Drawing for the job (mm, zero at the part's lowest x, y, z). A direction names the side the tool comes from. Round coordinates to 2 decimals unless told otherwise and drop trailing zeros. Loops run counter-clockwise (first coordinate to the right, second up) from the corner with the lowest first, then second, coordinate; pieces in that order, holes last. Notation, with made-up numbers: M 70,46.5 L 113,46.5 A18 ccw 113,51.5 Z; hole C 87,56.5 d11. An arc over 180 degrees is marked long. Use a Markdown table: item, result. Add a question column.
Q1. Probe line 1 (Y direction, x = 60.5, z = 3.75) (1 decimal); line 2 (X direction, y = 74, z = 5) (1 decimal); line 3 (Y direction, x = 13.5, z = 5.5). List the from-to ranges inside material, lowest first. Write a range as from..to.
Q2. Cut at A-A (x = 36). Give the cut face in (y, z) (1 decimal), plus the area to 3 significant figures.
Q3. Pin check, flat tips, straight feed: pin 1 (3 mm diameter, centred on y = 59, z = 7, fed in from -X) (1 decimal); pin 2 (5 mm diameter, centred on x = 60.325, y = 40.64, fed in from -Z); pin 3 (5 mm diameter, centred on x = 7, z = 3.5, fed in from +Y); pin 4 (3 mm diameter, centred on x = 13.5, z = 5.5, fed in from +Y). Stop position of each tip, or through.
Q4. Tool access for the marked faces 1, 2 and 3: list every direction of +Z, -Z, +X, -X, +Y, -Y with a clear straight run to the whole face (end or side of a thin tool).
Q5. Cut at B-B (z = 8). State how many separate pieces and enclosed holes the cut face has, plus the area to 3 significant figures.
Q6. Mould opens along X. For the marked faces 4, 5 and 6 say: +X half, -X half, draft (parallel to the pull), parting line (faces both ways), or undercut.
Q7. Cut at C-C (y = 64.5). Give the cut face in (x, z) (1 decimal).
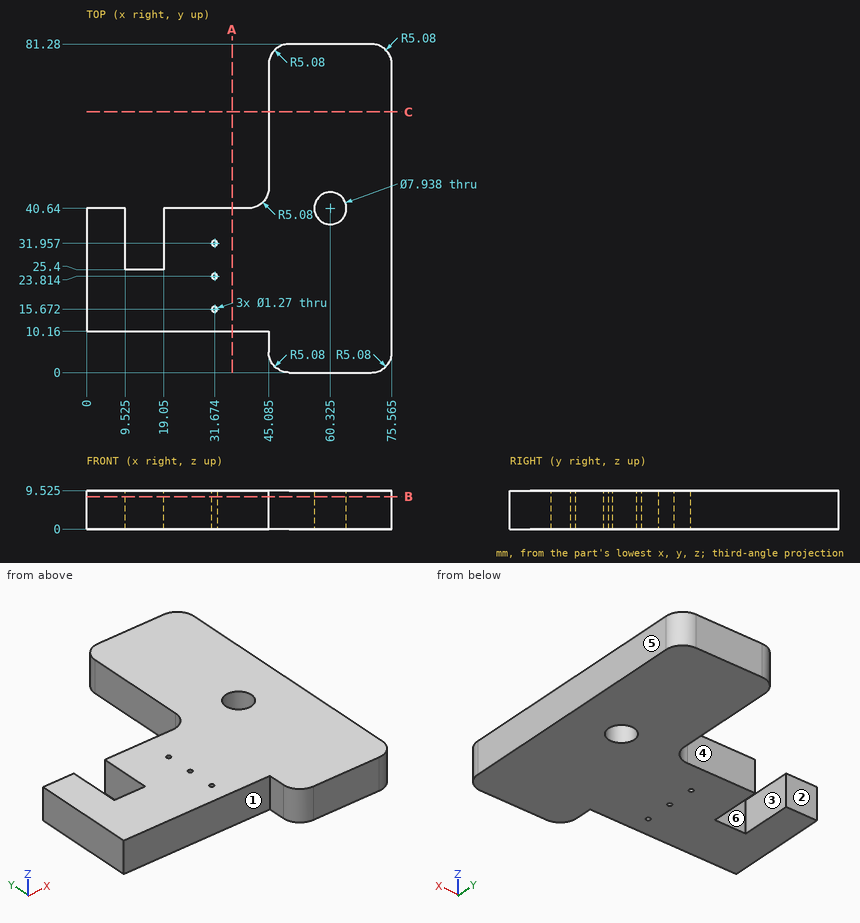
Checked values:
| question | item | result |
|---|---|---|
| 1 | line 1 | y = 0..36.7, 44.6..81.3 |
| 1 | line 2 | x = 45.1..75.6 |
| 1 | line 3 | y = 10.16..25.4 |
| 2 | outline | M 10.2,0 L 40.6,0 L 40.6,9.5 L 10.2,9.5 Z |
| 2 | area | 290 mm^2 |
| 3 | pin 1 | stops at x = 45.1 |
| 3 | pin 2 | passes through |
| 3 | pin 3 | stops at y = 40.64 |
| 3 | pin 4 | stops at y = 25.4 |
| 4 | face 1 | +Z, -Z, -X, -Y |
| 4 | face 2 | +Z, -Z, -X, +Y |
| 4 | face 3 | +Z, -Z, +Y |
| 5 | separate pieces | 1 |
| 5 | enclosed holes | 4 |
| 5 | area | 3,640 mm^2 |
| 6 | face 4 | draft |
| 6 | face 5 | +X half |
| 6 | face 6 | undercut |
| 7 | outline | M 45.1,0 L 75.6,0 L 75.6,9.5 L 45.1,9.5 Z |
